```python
from build123d import *

# Parameters (mm, degrees)
SKETCH5_W                      = 301.625
SKETCH5_H                      = 1.5875
BASE_FLANGE1_DEPTH             = 381
SKETCH10_W                     = 11.1125
SKETCH10_H                     = 12.7
BOSS_EXTRUDE1_DEPTH            = 1.5875
EDGE_FLANGE1_STRIP_W           = 12.7
EDGE_FLANGE1_STRIP_H           = 1.5875
EDGE_FLANGE1_STRIP_CUT_DEPTH   = 368.3
EDGE_FLANGE1_STRIP_2_W         = 12.7
EDGE_FLANGE1_STRIP_2_H         = 1.5875
EDGE_FLANGE1_STRIP_CUT_2_DEPTH = 368.3
EDGE_FLANGE1_DEPTH             = 368.3
EDGE_FLANGE1_BEND_DEPTH        = 368.3
CUT_EXTRUDE1_START             = -25.4
CUT_EXTRUDE1_DEPTH             = 342.9
EDGE_FLANGE2_STRIP_W           = 11.43
EDGE_FLANGE2_STRIP_H           = 1.5875
EDGE_FLANGE2_STRIP_CUT_DEPTH   = 25.4
EDGE_FLANGE2_DEPTH             = 25.4
EDGE_FLANGE3_STRIP_W           = 11.43
EDGE_FLANGE3_STRIP_H           = 1.5875
EDGE_FLANGE3_STRIP_CUT_DEPTH   = 25.4
EDGE_FLANGE3_DEPTH             = 25.4
FILLET1_R                      = 8
FILLET2_R                      = 3.175
SKETCH30_W                     = 4
SKETCH30_H                     = 1.5875
CUT_EXTRUDE9_DEPTH             = 4
SKETCH31_W                     = 4
SKETCH31_H                     = 1.5875
CUT_EXTRUDE10_DEPTH            = 4
FILLET4_R                      = 1.5


# Sheet-metal steps are written as plain solids
with BuildPart() as part:
    # Sketch5 → Base-Flange1 (new body)
    with BuildSketch(Plane.XY):
        with Locations((0, -0.79375)):
            Rectangle(SKETCH5_W, SKETCH5_H)
    extrude(amount=BASE_FLANGE1_DEPTH)

    # Sketch10 → Boss-Extrude1 (add)
    with BuildSketch(Plane(origin=(0, 0, 0), x_dir=(1, 0, 0), z_dir=(0, 1, 0))):
        with Locations((-156.36875, -6.35)):
            Rectangle(SKETCH10_W, SKETCH10_H)
        with Locations((156.36875, -6.35)):
            Rectangle(SKETCH10_W, SKETCH10_H)
    extrude(amount=-BOSS_EXTRUDE1_DEPTH)

    # Edge-Flange1 strip (across the edge) → Edge-Flange1 strip cut (cut)
    with BuildSketch(Plane(origin=(150.8125, -1.5875, 12.7), x_dir=(-1, 0, 0), z_dir=(0, 0, 1))):
        with Locations((-1.5875, -0.79375)):
            Rectangle(EDGE_FLANGE1_STRIP_W, EDGE_FLANGE1_STRIP_H)
    extrude(amount=EDGE_FLANGE1_STRIP_CUT_DEPTH, mode=Mode.SUBTRACT)

    # Edge-Flange1 strip 2 (across the edge) → Edge-Flange1 strip cut 2 (cut)
    with BuildSketch(Plane(origin=(-150.8125, -1.5875, 381), x_dir=(1, 0, 0), z_dir=(0, 0, -1))):
        with Locations((-1.5875, -0.79375)):
            Rectangle(EDGE_FLANGE1_STRIP_2_W, EDGE_FLANGE1_STRIP_2_H)
    extrude(amount=EDGE_FLANGE1_STRIP_CUT_2_DEPTH, mode=Mode.SUBTRACT)

    # Edge-Flange1 section (across the edge) → Edge-Flange1 (add)
    with BuildSketch(Plane(origin=(150.8125, -1.5875, 12.7), x_dir=(-1, 0, 0), z_dir=(0, 0, 1))):
        with BuildLine():
            Line((0, 3.175), (0, 23.8125))
            Line((0, 23.8125), (1.5875, 23.8125))
            Line((1.5875, 23.8125), (1.5875, 3.175))
            ThreePointArc((1.5875, 3.175), (2.51743597, 0.92993597), (4.7625, 0))
            Line((4.7625, 0), (4.7625, -1.5875))
            ThreePointArc((4.7625, -1.5875), (1.394903955, -0.192596045), (0, 3.175))
        make_face()
    extrude(amount=EDGE_FLANGE1_DEPTH)

    # Edge-Flange1 section 2 (across the edge) → Edge-Flange1 bend (add)
    with BuildSketch(Plane(origin=(-150.8125, -1.5875, 381), x_dir=(1, 0, 0), z_dir=(0, 0, -1))):
        with BuildLine():
            Line((0, 3.175), (0, 23.8125))
            Line((0, 23.8125), (1.5875, 23.8125))
            Line((1.5875, 23.8125), (1.5875, 3.175))
            ThreePointArc((1.5875, 3.175), (2.51743597, 0.92993597), (4.7625, 0))
            Line((4.7625, 0), (4.7625, -1.5875))
            ThreePointArc((4.7625, -1.5875), (1.394903955, -0.192596045), (0, 3.175))
        make_face()
    extrude(amount=EDGE_FLANGE1_BEND_DEPTH)

    # Sketch20 → Cut-Extrude1 (cut)
    with BuildSketch(Plane.XY.offset(381).offset(CUT_EXTRUDE1_START)):
        with BuildLine():
            Line((-150.8125, -4.7625), (-150.8125, -25.4))
            Line((-150.8125, -25.4), (-149.225, -25.4))
            Line((-149.225, -25.4), (-149.225, -4.7625))
            ThreePointArc((-149.225, -4.7625), (-148.29506403, -2.51743597), (-146.05, -1.5875))
            Line((-146.05, -1.5875), (-146.05, 0))
            ThreePointArc((-146.05, 0), (-149.417596045, -1.394903955), (-150.8125, -4.7625))
        make_face()
        with BuildLine():
            Line((149.225, -4.7625), (149.225, -25.4))
            Line((149.225, -25.4), (150.8125, -25.4))
            Line((150.8125, -25.4), (150.8125, -4.7625))
            ThreePointArc((150.8125, -4.7625), (149.417596045, -1.394903955), (146.05, 0))
            Line((146.05, 0), (146.05, -1.5875))
            ThreePointArc((146.05, -1.5875), (148.29506403, -2.51743597), (149.225, -4.7625))
        make_face()
    extrude(amount=-CUT_EXTRUDE1_DEPTH, mode=Mode.SUBTRACT)

    # Edge-Flange2 strip (across the edge) → Edge-Flange2 strip cut (cut)
    with BuildSketch(Plane(origin=(-150.8125, -25.4, 355.6), x_dir=(0, 1, 0), z_dir=(0, 0, 1))):
        with Locations((-1.5875, -0.79375)):
            Rectangle(EDGE_FLANGE2_STRIP_W, EDGE_FLANGE2_STRIP_H)
    extrude(amount=EDGE_FLANGE2_STRIP_CUT_DEPTH, mode=Mode.SUBTRACT)

    # Edge-Flange2 section (across the edge) → Edge-Flange2 (add)
    with BuildSketch(Plane(origin=(-150.8125, -25.4, 355.6), x_dir=(0, 1, 0), z_dir=(0, 0, 1))):
        with BuildLine():
            Line((0, 2.54), (0, 11.1125))
            Line((0, 11.1125), (1.5875, 11.1125))
            Line((1.5875, 11.1125), (1.5875, 2.54))
            ThreePointArc((1.5875, 2.54), (2.331448776, 0.743948776), (4.1275, 0))
            Line((4.1275, 0), (4.1275, -1.5875))
            ThreePointArc((4.1275, -1.5875), (1.208916761, -0.378583239), (0, 2.54))
        make_face()
    extrude(amount=EDGE_FLANGE2_DEPTH)

    # Edge-Flange3 strip (across the edge) → Edge-Flange3 strip cut (cut)
    with BuildSketch(Plane(origin=(150.8125, -25.4, 381), x_dir=(0, 1, 0), z_dir=(0, 0, -1))):
        with Locations((-1.5875, -0.79375)):
            Rectangle(EDGE_FLANGE3_STRIP_W, EDGE_FLANGE3_STRIP_H)
    extrude(amount=EDGE_FLANGE3_STRIP_CUT_DEPTH, mode=Mode.SUBTRACT)

    # Edge-Flange3 section (across the edge) → Edge-Flange3 (add)
    with BuildSketch(Plane(origin=(150.8125, -25.4, 381), x_dir=(0, 1, 0), z_dir=(0, 0, -1))):
        with BuildLine():
            Line((0, 2.54), (0, 11.1125))
            Line((0, 11.1125), (1.5875, 11.1125))
            Line((1.5875, 11.1125), (1.5875, 2.54))
            ThreePointArc((1.5875, 2.54), (2.331448776, 0.743948776), (4.1275, 0))
            Line((4.1275, 0), (4.1275, -1.5875))
            ThreePointArc((4.1275, -1.5875), (1.208916761, -0.378583239), (0, 2.54))
        make_face()
    extrude(amount=EDGE_FLANGE3_DEPTH)

    # Fillet1
    fillet1_edges = [part.edges().sort_by_distance(p)[0] for p in [
        (-146.05, -0.79375, 12.7),
        (146.05, -0.79375, 12.7),
    ]]
    fillet(fillet1_edges, radius=FILLET1_R)

    # Fillet2
    fillet2_edges = [part.edges().sort_by_distance(p)[0] for p in [
        (-161.925, -0.79375, 12.7),
        (-161.925, -0.79375, 0),
        (-161.925, -24.60625, 355.6),
        (-161.925, -24.60625, 381),
        (161.925, -24.60625, 381),
        (161.925, -24.60625, 355.6),
        (161.925, -0.79375, 0),
        (161.925, -0.79375, 12.7),
    ]]
    fillet(fillet2_edges, radius=FILLET2_R)

    # Sketch30 → Cut-Extrude9 (cut)
    with BuildSketch(Plane.ZY.offset(146.05)):
        with Locations((353.6, -0.79375)):
            Rectangle(SKETCH30_W, SKETCH30_H)
    extrude(amount=-CUT_EXTRUDE9_DEPTH, mode=Mode.SUBTRACT)

    # Sketch31 → Cut-Extrude10 (cut)
    with BuildSketch(Plane(origin=(146.05, 0, 0), x_dir=(0, 0, -1), z_dir=(1, 0, 0))):
        with Locations((-353.6, -0.79375)):
            Rectangle(SKETCH31_W, SKETCH31_H)
    extrude(amount=-CUT_EXTRUDE10_DEPTH, mode=Mode.SUBTRACT)

    # Fillet4
    fillet4_edges = [part.edges().sort_by_distance(p)[0] for p in [
        (-146.05, -0.79375, 351.6),
        (-142.05, -0.79375, 351.6),
        (-142.05, -0.79375, 355.6),
        (146.05, -0.79375, 351.6),
        (142.05, -0.79375, 351.6),
        (142.05, -0.79375, 355.6),
    ]]
    fillet(fillet4_edges, radius=FILLET4_R)


solid = part.part
```
Work out the finished part from the listing and answer in its coordinate system (mm). A direction names the side the tool comes from. Coordinates: 2 decimals unless noted, no trailing zeros. Loops run counter-clockwise (first coordinate to the right, second up) from the corner with the lowest first, then second, coordinate; pieces in that order, holes last.
1) Section B-B (z = 346) is taken. Give the vertices of the cut face in (x, y), plus the area to 3 significant figures.
Results:
outline: (-146.05, -1.59) - (146.05, -1.59) - (146.05, 0) - (-146.05, 0) - close
area: 464 mm2
2) Section C-C (x = -2) is taken. Give the vertices of the cut face in (y, z).
Results:
outline: (-1.59, 0) - (0, 0) - (0, 381) - (-1.59, 381) - close
3) Consider probe 1 along Y at (x, z) = (-87, 345). Determine where the line is inside the solid, lowest interval first.
Results:
probe 1: y = -1.59 to 0
4) For a pull along Z with two mould halves and no side action, classify faces 1 (the flat face through (1, -1, 381)), 2 (the flat face through (150.6, -13.7, 355.6)), 3 (the flat face through (-158, -23.812, 368)) as +Z half, -Z half, draft (parallel to the pull), parting line (faces both ways), or undercut.
Results:
face 1: +Z half
face 2: undercut
face 3: draft
5) For faces 4 (the cylindrical face through (-148.456, -0.783, 14.981)), 5 (the flat face through (-150.812, -13, 368)), 6 (the flat face through (-149.225, -13, 368)), 7 (the cylindrical face through (148.331, -0.805, 15.106)), determine the directions among +Z, -Z, +X, -X, +Y, -Y from which every point of the face is accessible in a straight line to the end or side of a thin tool.
Results:
face 4: -X, +Y, -Y
face 5: +Z, -Z, -X, +Y
face 6: +Z, -Z, -Y
face 7: +X, +Y, -Y
6) Flat-ended cylindrical pins translate along their axes: pin 1 (10 mm diameter, centred on x = 24, y = -10, fed in from -Z); pin 2 (2 mm diameter, centred on x = 73.5, z = 56.5, fed in from -Y); pin 3 (4.5 mm diameter, centred on x = 151, y = -14.5, fed in from -Z); pin 4 (0.8 mm diameter, centred on y = -1, z = 354, fed in from -X). Find the tip coordinate at first contact, or state that the pin passes through.
Results:
pin 1: passes through
pin 2: stops at y = -1.59
pin 3: stops at z = 355.6
pin 4: stops at x = -142.08
7) Section A-A (y = -15) is taken. Give the vertices of the cut face in (x, z) (1 decimal).
Results:
outline: (-150.8, 355.6) - (-149.2, 355.6) - (-149.2, 381) - (-150.8, 381) - close; (149.2, 355.6) - (150.8, 355.6) - (150.8, 381) - (149.2, 381) - close
